Autodesk Inventor part; units mm, degrees
ref_plane "YZ Plane" through (0, 0, 0) normal (1, 0, 0) x (0, 1, 0)
ref_plane "XZ Plane" through (0, 0, 0) normal (0, 1, 0) x (-1, 0, 0)
ref_plane "XY Plane" through (0, 0, 0) normal (0, 0, 1) x (1, 0, 0)
ref_plane "Work Plane1" through (118.9518, 9.9874, -13.1749) normal (0.4728584, -0.8811384, 0) x (0, 0, -1)
sketch "Sketch1" plane through (118.9518, 9.9874, -13.1749) normal (0.4728584, -0.8811384, 0) x (0, 0, -1)
  line L0 (-16.5984, 5.5392) -> (-16.5984, 5.9228)
  line L1 (-1.2281, -14.4596) -> (-31.7652, -14.4596) construction
  line L2 (-16.5984, 11.5008) -> (-16.5984, -0.9971)
  line L3 (-15.5984, -2) -> (-12.5984, -2)
  line L4 (-16.5984, 2) -> (-12.5984, 2)
  line L5 (-16.5984, -2.6601) -> (-27.5984, -2.6601)
  line L6 (-27.5984, -2.6601) -> (-30.5984, -5.6601)
  line L7 (-30.5984, -5.6601) -> (-30.5984, -8.4596)
  line L8 (-30.5984, -8.4596) -> (-30.5984, -20.4596)
  line L9 (-30.5984, -20.4596) -> (-34.5984, -20.4596)
  line L10 (-34.5984, -20.4596) -> (-42.5984, -12.4596)
  line L11 (-42.5984, -12.4596) -> (-42.5984, -2.0772)
  line L12 (-42.5984, -2.0772) -> (-34.5984, 5.9228)
  line L13 (-34.5984, 5.9228) -> (-16.5984, 5.9228)
  line L14 (-16.5984, 0.8574) -> (-16.5984, 5.9228)
  line L15 (-16.5984, 3.3399) -> (-48.439, 3.3399) construction
  line L16 (-16.5984, -0.9971) -> (-16.5984, -2.6601)
  line L17 (-16.5984, -0.0772) -> (-40.5984, -0.0772) construction
  line L18 (-40.5984, -0.0772) -> (-40.5984, -14.4596) construction
  line L19 (-16.5984, -0.0772) -> (-40.5984, -0.0772)
  line L20 (-19.5984, -2.6601) -> (-17.0984, -2.6601)
  point P0 (-13.1749, -109.5356)
  point P1 (-16.5984, 0.8574)
  dimension "d25" = 135
  dimension "d26" = 4
  dimension "d27" = 6
  dimension "d28" = 2.5829
  dimension "d29" = 6
  dimension "d31" = 12
  dimension "d40" = 3
  dimension "d42" = 26
  dimension "d45" = 0
  dimension "d50" = 8
  dimension "d62" = 0
extrude "Extrusion1" add sketch "Sketch1" along normal blind 1.5
sketch "Sketch2" plane through (119.6611, 8.6657, -13.1749) normal (0.4728584, -0.8811384, 0) x (0.8811384, 0.4728584, 0)
  line L0 (-2.0772, 42.5984) -> (-12.4596, 42.5984)
  line L1 (-12.4596, 42.5984) -> (-20.4596, 34.5984)
  line L2 (-20.4596, 34.5984) -> (-20.4596, 30.5984)
  line L3 (-20.4596, 30.5984) -> (-5.6601, 30.5984)
  line L4 (-5.6601, 30.5984) -> (-2.6601, 27.5984)
  line L5 (-2.6601, 27.5984) -> (-2.6601, 16.5984)
  line L6 (5.9228, 16.5984) -> (5.9228, 34.5984)
  line L7 (5.9228, 34.5984) -> (-2.0772, 42.5984)
  line L8 (-2.6601, 16.5984) -> (5.9228, 16.5984)
  line L9 (-11.8383, 41.0984) -> (-2.6985, 41.0984)
  line L10 (-2.6985, 41.0984) -> (4.4228, 33.9771)
  line L11 (4.4228, 33.9771) -> (4.4228, 18.0984)
  line L12 (4.4228, 18.0984) -> (-0.9902, 18.0984)
  line L13 (-0.9902, 18.0984) -> (-1.1601, 18.0962)
  line L14 (-1.1601, 18.0962) -> (-1.1601, 28.2197)
  line L15 (-1.1601, 28.2197) -> (-5.0388, 32.0984)
  line L16 (-5.0388, 32.0984) -> (-8.9884, 32.0984)
  line L17 (-8.9884, 32.0984) -> (-9.9596, 32.0984)
  line L18 (-9.9596, 32.0984) -> (-18.9596, 32.0984)
  line L19 (-18.9596, 32.0984) -> (-18.9596, 33.9771)
  line L20 (-18.9596, 33.9771) -> (-11.8383, 41.0984)
  point P0 (-109.5356, 13.1749)
  point P1 (-0.7471, 18.0984)
  dimension "d41" = 1.5
  dimension "d63" = 1.5
extrude "Extrusion2" [suppressed]
sketch "Sketch3" plane through (103.5006, 1.6956, 17.4235) normal (0, 0, -1) x (-0.8811384, -0.4728584, 0)
  circle A0 centre (-2.8052, -7.75) radius 4.5
  line L0 (3.1948, 0) -> (-8.8052, 0)
  line L1 (-8.8052, 0) -> (-8.8052, -15.5)
  line L2 (3.1948, -15.5) -> (-8.8052, -15.5)
  line L3 (3.1948, 0) -> (3.1948, -15.5)
  point P0 (92.0001, 47.4471)
extrude "Extrusion3" cut sketch "Sketch3" against normal blind 1.5 contours A0
sketch "Sketch8" plane through (119.7213, 8.698, 3.4235) normal (0, 0, 1) x (0.8811384, 0.4728584, 0)
  circle A0 centre (-19.1075, 3.6497) radius 1.4001
  circle A1 centre (-14.1578, 7.8923) radius 2
  circle A2 centre (-14.1578, 7.8923) radius 3.3708
  point P0 (-109.604, 48.9471)
extrude "Extrusion8" cut sketch "Sketch8" along normal mid plane 14 contours A1 | A2
sketch "Sketch9" plane through (118.7885, 8.1974, 4.9235) normal (0, 0, 1) x (0.8811384, 0.4728584, 0)
  circle A0 centre (0.9902, -6.25) radius 1.352
  circle A1 centre (0.9902, -6.25) radius 2.6601
  point P0 (-108.5454, 48.9471)
extrude "Extrusion9" [suppressed]
ref_plane "Arbeitsebene3" through (124.1706, 12.788, 7.4235) normal (0, 0, -1) x (-0.8811384, -0.4728584, 0)
sketch "Skizze13" plane through (124.1706, 12.788, 7.4235) normal (0, 0, -1) x (-0.8811384, -0.4728584, 0)
  line L0 (0, 0) -> (0, -1.5)
  circle A0 centre (-2.8278, -9.3645) radius 1.1933
  line L1 (8.5829, 0) -> (0, 0)
  line L2 (0, 0) -> (0, -15.5)
  line L3 (0, -15.5) -> (-6.5, -15.5)
  line L4 (-6.5, -15.5) -> (-6.5, 0)
  line L5 (-6.5, 0) -> (0, 0)
  circle A1 centre (-2.8278, -9.3645) radius 1.6
  circle A2 centre (-2.8278, -9.3645) radius 1.75
  point P0 (115.4584, 47.4471)
  point P1 (-2.8531, -15.3156)
  dimension "d58" = 6.5
  dimension "d66" = 3.5
extrude "Extrusion13" [suppressed]
fillet "Rundung1" radius 2 7 edges at (124.5253, 12.1272, 21.4235) (108.3278, 3.4349, 29.4235) (101.2787, -0.348, 21.4235) (101.2787, -0.348, 17.4235) (114.3191, 6.6501, 17.4235) (116.9625, 8.0687, 14.4235) (117.4762, 8.3443, 29.4235)
sketch "Skizze14" plane through (118.9518, 9.9874, -13.1749) normal (-0.4728584, 0.8811384, 0) x (0.8811384, 0.4728584, 0)
  arc A0 (3.8371, -34.5629) -> (4.4228, -33.1487) centre (2.4228, -33.1487) ccw
  line L0 (3.8371, -34.5629) -> (-2.1127, -40.5126)
  arc A1 (-3.5269, -41.0984) -> (-2.1127, -40.5126) centre (-3.5269, -39.0984) ccw
  line L1 (-3.5269, -41.0984) -> (-11.0098, -41.0984)
  arc A2 (-12.4241, -40.5126) -> (-11.0098, -41.0984) centre (-11.0098, -39.0984) ccw
  line L2 (-12.4241, -40.5126) -> (-17.4241, -35.5126)
  arc A3 (-16.0098, -32.0984) -> (-17.4241, -35.5126) centre (-16.0098, -34.0984) ccw
  line L3 (-16.0098, -32.0984) -> (-5.4542, -32.0984)
  arc A4 (-5.4542, -32.0984) -> (-4.04, -31.5126) centre (-5.4542, -30.0984) ccw
  line L4 (-4.04, -31.5126) -> (-1.3329, -28.8055)
  arc A5 (-1.3329, -28.8055) -> (-0.7471, -27.3913) centre (-2.7471, -27.3913) ccw
  line L5 (-0.7471, -27.3913) -> (-0.7471, -18.0984)
  line L6 (-0.7471, -18.0984) -> (4.4228, -18.0984)
  line L7 (4.4228, -18.0984) -> (4.4228, -33.1487)
  point P0 (-109.5356, -13.1749)
extrude "Extrusion14" cut sketch "Skizze14" against normal blind 10
properties part number "Matchboxscope_Lightperiscope_long_V0"
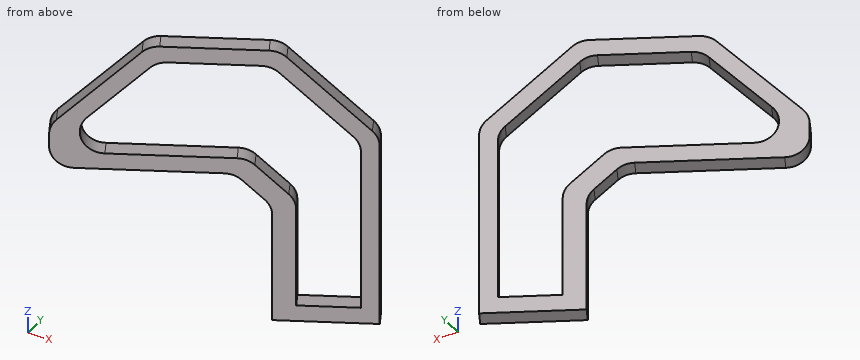
For this review, take the finished solid that the model builds, in its own axes (mm). Give positions to 0.01 mm unless a question says otherwise; leave off trailing zeros. Order: outer loops, then holes, each group sorted by start corner. A loop starts at its lowest first (then second) coordinate and runs counter-clockwise, first axis right, second up.
1) Take a section at A-A (z = 23). Give the boundary of the cut face in (x, y).
2) Insertion check: pin 1 (1 mm diameter, centred on x = 112, y = 8, fed in from +Z); pin 2 (3 mm diameter, centred on x = 121.5, y = 11, fed in from +Z); pin 3 (2 mm diameter, centred on x = 118.5, z = 10.5, fed in from +Y); pin 4 (4 mm diameter, centred on y = 6, z = 17.5, fed in from -X). Each pin has a flat end and moves straight along its axis. Give the tip position at first contact, or say it passes through.
3) Wall thickness on line 1 (Z direction, x = 117.25, y = 8.75); line 2 (Z direction, x = 118.75, y = 9.25); line 3 (X direction, y = 0, z = 22.75): over which ranges is each line inside the solid? List them lowest first.
4) Take a section at B-B (x = 120.5). Give the boundary of the cut face in (y, z).
Derived:
1. outline: (102.31, 1.06) - (103.02, -0.26) - (104.89, 0.74) - (104.18, 2.06) - close; (120.91, 11.04) - (121.62, 9.72) - (123.49, 10.72) - (122.78, 12.04) - close
2. pin 1: passes through
2. pin 2: stops at z = 26.12
2. pin 3: stops at y = 9.63
2. pin 4: stops at x = 107.79
3. line 1: z = 3.42 to 16.38, 27.31 to 29.25
3. line 2: z = 3.42 to 4.92, 25.75 to 27.87
3. line 3: x = 102.6 to 103.51
4. outline: (9.12, 3.42) - (10.82, 3.42) - (10.82, 4.92) - (9.12, 4.92) - close; (9.12, 24.27) - (10.82, 23.47) - (10.82, 25.59) - (9.12, 26.39) - close
